from build123d import *

# Parameters (mm, degrees)
EXTRUDE_2_DEPTH     = 15
SKETCH_2_R          = 2.62067407
CUT_EXTRUDE_1_DEPTH = 30
CUT_EXTRUDE_2_DEPTH = 3
SKETCH_5_R          = 10.35
CUT_EXTRUDE_3_DEPTH = 3
SKETCH_6_R          = 1.75
CUT_EXTRUDE_4_DEPTH = 73
FILLET_1_R          = 7
FILLET_2_R          = 15
CUT_EXTRUDE_5_DEPTH = 80


with BuildPart() as part:
    # 草图1 → 拉伸-薄壁2 (new, symmetric)
    with BuildSketch(Plane.XY):
        Polygon((29.774038515, -24.3), (29.774038515, 97.117302362), (0, 97.117302362), (-29.774038515, 97.117302362), (-29.774038515, -24.3), (-25.774038515, -24.3), (-25.774038515, 93.117302362), (0, 93.117302362), (25.774038515, 93.117302362), (25.774038515, -24.3), align=None)
    extrude(amount=EXTRUDE_2_DEPTH, both=True)

    # 草图2 → 切除-拉伸1 (cut)
    with BuildSketch(Plane(origin=(0, 97.117302362, 0), x_dir=(1, 0, 0), z_dir=(0, 1, 0))):
        with Locations(Location((-15, 0, 0), (0, 0, 270))):
            Circle(SKETCH_2_R)
        with Locations(Location((15, 0, 0), (0, 0, 270))):
            Circle(SKETCH_2_R)
    extrude(amount=-CUT_EXTRUDE_1_DEPTH, mode=Mode.SUBTRACT)

    # 草图4 → 切除-拉伸2 (cut)
    with BuildSketch(Plane.ZY.offset(-25.774038515)):
        with BuildLine():
            Line((-2.776256892, 22.163864907), (-5.090172263, 4.508896355))
            ThreePointArc((-5.090172263, 4.508896355), (-6.8, 0), (-5.090172263, -4.508896355))
            Line((-5.090172263, -4.508896355), (-2.776256892, -22.163864907))
            ThreePointArc((-2.776256892, -22.163864907), (0, -24.6), (2.776256892, -22.163864907))
            Line((2.776256892, -22.163864907), (5.090172263, -4.508896355))
            ThreePointArc((5.090172263, -4.508896355), (6.8, 0), (5.090172263, 4.508896355))
            Line((5.090172263, 4.508896355), (2.776256892, 22.163864907))
            ThreePointArc((2.776256892, 22.163864907), (0, 24.6), (-2.776256892, 22.163864907))
        make_face()
    extrude(amount=-CUT_EXTRUDE_2_DEPTH, mode=Mode.SUBTRACT)

    # 草图5 → 切除-拉伸3 (cut)
    with BuildSketch(Plane(origin=(-25.774038515, 0, 0), x_dir=(0, 0, -1), z_dir=(1, 0, 0))):
        Circle(SKETCH_5_R)
    extrude(amount=-CUT_EXTRUDE_3_DEPTH, mode=Mode.SUBTRACT)

    # 草图6 → 切除-拉伸4 (cut)
    with BuildSketch(Plane.ZY.offset(29.774038515)):
        Circle(SKETCH_6_R)
    extrude(amount=-CUT_EXTRUDE_4_DEPTH, mode=Mode.SUBTRACT)

    # 圆角1
    fillet_1_edges = [part.edges().sort_by_distance(p)[0] for p in [
        (25.774038515, 93.117302362, 0),
        (-25.774038515, 93.117302362, 0),
    ]]
    fillet(fillet_1_edges, radius=FILLET_1_R)

    # 圆角2
    fillet_2_edges = [part.edges().sort_by_distance(p)[0] for p in [
        (27.774038515, -24.3, -15),
        (-27.774038515, -24.3, -15),
        (-27.774038515, -24.3, 15),
        (27.774038515, -24.3, 15),
    ]]
    fillet(fillet_2_edges, radius=FILLET_2_R - 0.0001)  # a hair under: the kernel refuses the full size

    # 草图7 → 切除-拉伸5 (cut)
    with BuildSketch(Plane.ZY.offset(29.774038515)):
        with BuildLine():
            ThreePointArc((15, 0), (0, -15), (-15, 0))
            Line((-15, 0), (-15, -9.3))
            ThreePointArc((-15, -9.3), (-10.606601718, -19.906601718), (0, -24.3))
            ThreePointArc((0, -24.3), (10.606601718, -19.906601718), (15, -9.3))
            Line((15, -9.3), (15, 0))
        make_face()
    extrude(amount=-CUT_EXTRUDE_5_DEPTH, mode=Mode.SUBTRACT)


with BuildPart() as cut_extrude_5_kept_piece:
    # of the separate pieces the step leaves, the one the design keeps (cut_extrude_5_pieces_kept)
    add(part.part.solids().sort_by_distance((-29.774038515, 0, -15))[0])


solid = cut_extrude_5_kept_piece.part
Verification items for the finished model (mm, model axes). A direction names the side the tool comes from. Coordinates: 2 decimals unless noted, no trailing zeros. Order: outer loops, then holes, each group sorted by start corner. A loop starts at its lowest first (then second) coordinate and runs counter-clockwise, first axis right, second up.
1. Release check for a two-part mould opening along X. For faces 5 (the face through (17.21, 95.15, 1.41)), 6 (the face through (29, -15, 0)), 7 (the face through (0, 93.117, 0)), 8 (the face through (-29.774, 42, 0)) record: +X half, -X half, draft (parallel to the pull), parting line (faces both ways), or undercut.
Results found:
face 5: undercut
face 6: draft
face 7: undercut
face 8: -X half
2. Go/stop test with flat-tipped pins: pin 1 Ø3 at (y, z) = (0, 0) entering from -X; pin 2 Ø1.5 at (x, z) = (10.5, -6) entering from -Y. Record where each tip stops, or that it passes through.
Results found:
pin 1: passes through
pin 2: stops at y = 93.12
3. Scan lines: line 1 (X direction, y = 94.65, z = 0); line 2 (X direction, y = 80, z = -2.75); line 3 (X direction, y = 2.5, z = -9.75). Record each from-to range of solid material in increasing order.
Results found:
line 1: x = -29.77 to -17.62, -12.38 to 12.38, 17.62 to 29.77
line 2: x = -29.77 to -25.77, 25.77 to 29.77
line 3: x = -29.77 to -28.77, 25.77 to 29.77
4. Sectioned sample at D-D, the plane x = -2.5. Record the cut outline in (y, z).
Results found:
outline: (93.12, -15) - (97.12, -15) - (97.12, 15) - (93.12, 15) - close
5. Sectioned sample at A-A, the plane y = 65. Record the cut outline in (x, z).
Results found:
outline: (-29.77, -15) - (-25.77, -15) - (-25.77, 15) - (-29.77, 15) - close; (25.77, -15) - (29.77, -15) - (29.77, 15) - (25.77, 15) - close
6. Set-up check for faces 1 (the face through (27.3, 24.6, 0.1)), 2 (the face through (27.25, 13.21, 3.95)), 3 (the face through (0, 97.117, 0)), 4 (the face through (-25.774, 35, 0)): record each of +Z, -Z, +X, -X, +Y, -Y from which the full face is reachable in a straight line by a thin tool's end or side.
Results found:
face 1: -Y
face 2: none
face 3: +Z, -Z, +X, -X, +Y
face 4: +Z, -Z, -Y
7. Sectioned sample at B-B, the plane z = 0. Give the number of separate pieces and of enclosed holes in the cut face, and give its area (3 significant figures).
Results found:
separate pieces: 5
enclosed holes: 0
area: 894 mm2
8. Sectioned sample at C-C, the plane x = 15. Record the cut outline in (y, z), and give its area (3 significant figures).
Results found:
outline: (93.12, -15) - (97.12, -15) - (97.12, -2.62) - (93.12, -2.62) - close; (93.12, 2.62) - (97.12, 2.62) - (97.12, 15) - (93.12, 15) - close
area: 99.0 mm2
